Autodesk Inventor part; units mm, degrees
ref_plane "YZ Plane" through (0, 0, 0) normal (1, 0, 0) x (0, 1, 0)
ref_plane "XZ Plane" through (0, 0, 0) normal (0, 1, 0) x (-1, 0, 0)
ref_plane "XY Plane" through (0, 0, 0) normal (0, 0, 1) x (1, 0, 0)
sketch "Sketch1" plane through (0, 0, 0) normal (0, 0, 1) x (1, 0, 0)
  arc A0 (-20.5392, 17.1146) -> (-21.125, 15.7004) centre (-19.125, 15.7004) ccw
  line L0 (-21.125, -15.7004) -> (-21.125, 15.7004)
  arc A1 (-21.125, -15.7004) -> (-20.5392, -17.1146) centre (-19.125, -15.7004) ccw
  line L1 (-20.5392, -17.1146) -> (-17.1146, -20.5392)
  arc A2 (-17.1146, -20.5392) -> (-15.7004, -21.125) centre (-15.7004, -19.125) ccw
  line L2 (15.7004, -21.125) -> (-15.7004, -21.125)
  arc A3 (15.7004, -21.125) -> (17.1146, -20.5392) centre (15.7004, -19.125) ccw
  line L3 (20.5392, -17.1146) -> (17.1146, -20.5392)
  arc A4 (20.5392, -17.1146) -> (21.125, -15.7004) centre (19.125, -15.7004) ccw
  line L4 (21.125, 15.7004) -> (21.125, -15.7004)
  arc A5 (21.125, 15.7004) -> (20.5392, 17.1146) centre (19.125, 15.7004) ccw
  line L5 (20.5392, 17.1146) -> (17.1146, 20.5392)
  arc A6 (17.1146, 20.5392) -> (15.7004, 21.125) centre (15.7004, 19.125) ccw
  line L6 (-15.7004, 21.125) -> (15.7004, 21.125)
  arc A7 (-15.7004, 21.125) -> (-17.1146, 20.5392) centre (-15.7004, 19.125) ccw
  line L7 (-20.5392, 17.1146) -> (-17.1146, 20.5392)
  circle A8 centre (0, 0) radius 16
  circle A9 centre (-15.875, -15.875) radius 1.625
  circle A10 centre (15.875, 15.875) radius 1.625
  circle A11 centre (-15.875, 15.875) radius 1.625
  circle A12 centre (15.875, -15.875) radius 1.625
  circle A13 centre (0, 0) radius 12
  circle A14 centre (-15.875, 15.875) radius 2
  circle A15 centre (15.875, 15.875) radius 2
  circle A16 centre (15.875, -15.875) radius 2
  circle A17 centre (-15.875, -15.875) radius 2
  point P0 (0, 0)
  dimension "d0" = 24
  dimension "d1" = 4
  dimension "d2" = 4
  dimension "d3" = 4
  dimension "d4" = 4
extrude "Extrusion1" add sketch "Sketch1" along normal blind 5 contours L7 A7 L6 A6 L5 A5 L4 A4 L3 A3 L2 A2 L1 A1 L0 A0 | A8
sketch "Sketch3" plane through (0, 0, 5) normal (0, 0, 1) x (1, 0, 0)
  line L0 (-15.7004, 21.125) -> (15.7004, 21.125)
  line L1 (15.7004, 21.125) -> (-46.125, 21.125)
  line L2 (-46.125, 21.125) -> (-46.125, 26.125)
  line L3 (-46.125, 26.125) -> (15.7004, 26.125)
  line L4 (15.7004, 26.125) -> (15.7004, 21.125)
  line L5 (-21.125, 15.7004) -> (-21.125, -15.7004)
  line L6 (-21.125, -15.7004) -> (-26.125, -15.7004)
  line L7 (-26.125, -15.7004) -> (-26.125, 46.125)
  line L8 (-26.125, 46.125) -> (-21.125, 46.125)
  line L9 (-21.125, 46.125) -> (-21.125, -15.7004)
  point P0 (0, 0)
  dimension "d11" = 5
  dimension "d12" = 5
  dimension "d13" = 20
  dimension "d14" = 20
extrude "Extrusion3" add sketch "Sketch3" against normal blind 40
sketch "Sketch4" plane through (0, 0, 5) normal (0, 0, 1) x (1, 0, 0)
  arc A0 (-15.7004, 21.125) -> (-17.1146, 20.5392) centre (-15.7004, 19.125) ccw
  line L0 (-17.1146, 20.5392) -> (-20.5392, 17.1146)
  arc A1 (-20.5392, 17.1146) -> (-21.125, 15.7004) centre (-19.125, 15.7004) ccw
  line L1 (-21.125, 21.125) -> (-21.125, 15.7004)
  line L2 (-15.7004, 21.125) -> (-21.125, 21.125)
  circle A2 centre (0, 0) radius 12
  circle A3 centre (-15.875, -15.875) radius 2
  circle A4 centre (15.875, -15.875) radius 2
  circle A5 centre (15.875, 15.875) radius 2
  circle A6 centre (-15.875, 15.875) radius 2
  line L3 (15.7004, 26.125) -> (15.7004, 21.125)
  line L4 (-21.125, 26.125) -> (15.7004, 26.125)
  line L5 (-21.125, 46.125) -> (-21.125, 26.125)
  line L6 (-26.125, 46.125) -> (-21.125, 46.125)
  line L7 (-26.125, 26.125) -> (-26.125, 46.125)
  line L8 (-46.125, 26.125) -> (-26.125, 26.125)
  line L9 (-46.125, 21.125) -> (-46.125, 26.125)
  line L10 (-26.125, 21.125) -> (-46.125, 21.125)
  line L11 (-26.125, -15.7004) -> (-26.125, 21.125)
  line L12 (-21.125, -15.7004) -> (-26.125, -15.7004)
  arc A7 (-21.125, -15.7004) -> (-20.5392, -17.1146) centre (-19.125, -15.7004) ccw
  line L13 (-20.5392, -17.1146) -> (-17.1146, -20.5392)
  arc A8 (-17.1146, -20.5392) -> (-15.7004, -21.125) centre (-15.7004, -19.125) ccw
  line L14 (-15.7004, -21.125) -> (15.7004, -21.125)
  arc A9 (15.7004, -21.125) -> (17.1146, -20.5392) centre (15.7004, -19.125) ccw
  line L15 (17.1146, -20.5392) -> (20.5392, -17.1146)
  arc A10 (20.5392, -17.1146) -> (21.125, -15.7004) centre (19.125, -15.7004) ccw
  line L16 (21.125, -15.7004) -> (21.125, 15.7004)
  arc A11 (21.125, 15.7004) -> (20.5392, 17.1146) centre (19.125, 15.7004) ccw
  line L17 (20.5392, 17.1146) -> (17.1146, 20.5392)
  arc A12 (17.1146, 20.5392) -> (15.7004, 21.125) centre (15.7004, 19.125) ccw
  point P0 (0, 0)
extrude "Extrusion4" add sketch "Sketch4" against normal blind 5 contours A0 L0 A1 L1 L2
sketch "Sketch11" plane through (0, 0, 5) normal (0, 0, 1) x (1, 0, 0)
  line L0 (-26.125, 26.125) -> (-26.125, 46.125)
  line L1 (-26.125, 26.125) -> (-13.6996, 26.125)
  line L2 (-13.6996, 26.125) -> (-13.6996, 46.125)
  line L3 (-13.6996, 46.125) -> (-26.125, 46.125)
  line L4 (-26.125, 46.125) -> (-26.125, 26.125)
  line L5 (-46.125, 21.125) -> (-46.125, 26.125)
  line L6 (-46.125, 26.125) -> (-26.125, 26.125)
  line L7 (-26.125, 26.125) -> (-26.125, 13.3287)
  line L8 (-26.125, 13.3287) -> (-46.125, 13.3287)
  line L9 (-46.125, 13.3287) -> (-46.125, 26.125)
  point P0 (0, 0)
extrude "Extrusion9" cut sketch "Sketch11" against normal blind 20
sketch "Sketch7" plane through (0, 0, -35) normal (0, 0, -1) x (-1, 0, 0)
  line L0 (21.625, 21.625) -> (-23.2924, 21.625)
  line L1 (-23.2924, 21.625) -> (-23.2924, -21.9013)
  line L2 (-23.2924, -21.9013) -> (21.625, -21.9013)
  line L3 (21.625, -21.9013) -> (21.625, 21.625)
  line L4 (-15.7004, 21.125) -> (21.125, 21.125)
  line L5 (21.125, 21.125) -> (21.125, -15.7004)
  point P0 (0, 0)
  dimension "d35" = 0.5
  dimension "d36" = 0.5
extrude "Extrusion7" cut sketch "Sketch7" against normal blind 35
sketch "Sketch12" plane through (0, 0, -35) normal (0, 0, -1) x (-1, 0, 0)
  line L0 (46.125, 21.125) -> (46.125, 26.125)
  line L1 (26.125, 26.125) -> (-15.7004, 26.125)
  line L2 (46.125, 21.125) -> (21.6284, 21.125)
  line L3 (21.6284, 21.125) -> (21.6284, 26.125)
  line L4 (21.6284, 26.125) -> (46.125, 26.125)
  line L5 (46.125, 26.125) -> (46.125, 21.125)
  line L6 (26.125, 46.125) -> (21.125, 46.125)
  line L7 (-15.7004, 21.625) -> (21.625, 21.625)
  line L8 (26.125, 46.125) -> (21.125, 46.125)
  line L9 (21.125, 46.125) -> (21.125, 21.625)
  line L10 (21.125, 21.625) -> (26.125, 21.625)
  line L11 (26.125, 21.625) -> (26.125, 46.125)
  point P0 (0, 0)
  point P1 (21.125, 26.125)
  dimension "d54" = 5
  dimension "d55" = 5
  dimension "d56" = 4.5
  dimension "d57" = 0.5
extrude "Extrusion10" add sketch "Sketch12" along normal blind 20 contours L2 L3 L10 L11 L4 L0 | L11 L10 L3 L1 | L1 L9 L6 L11
sketch "Sketch13" plane through (-46.125, 21.125, -15) normal (0, -1, 0) x (1, 0, 0)
  circle A0 centre (10, -30) radius 2.5
  circle A1 centre (10, -10) radius 2.5
  line L0 (24.4966, -40) -> (0, -40)
  line L1 (0, 0) -> (0, -40)
  point P0 (46.125, 15)
  dimension "d60" = 10
  dimension "d61" = 10
  dimension "d62" = 5
  dimension "d63" = 5
  dimension "d64" = 20
  dimension "d65" = 10
extrude "Extrusion11" cut sketch "Sketch13" against normal blind 20
sketch "Sketch14" plane through (-26.125, 26.125, -15) normal (-1, 0, 0) x (0, 0, 1)
  circle A0 centre (-10, 10) radius 2.5
  circle A1 centre (-30, 10) radius 2.5
  line L0 (0, 0) -> (0, 20)
  line L1 (0, 20) -> (-40, 20)
  point P0 (15, -26.125)
  dimension "d68" = 10
  dimension "d69" = 10
  dimension "d70" = 20
  dimension "d71" = 10
  dimension "d72" = 5
  dimension "d73" = 5
extrude "Extrusion12" cut sketch "Sketch14" against normal blind 20
equation "\"d36\" = d35"
properties part number "StepperXYHolder"
Design review of the part built by this model. Coordinates are the model's own, in mm. A direction names the side the tool comes from. Round coordinates to 2 decimals unless told otherwise and drop trailing zeros. Order: outer loops, then holes, each group sorted by start corner. A loop starts at its lowest first (then second) coordinate and runs counter-clockwise, first axis right, second up.
1) Clearance check with flat-ended pins moving along their axes: pin 1 Ø3 at (y, z) = (6, -30) entering from -X (3 decimals); pin 2 Ø1.5 at (y, z) = (22.5, -10.5) entering from +X; pin 3 Ø6 at (x, z) = (-38.5, -26.5) entering from +Y (3 decimals); pin 4 Ø5 at (x, y) = (-34.5, 31) entering from -Z. State where each tip first meets the part, or that it passes through.
The answers:
pin 1: stops at x = -26.125
pin 2: stops at x = 15.7
pin 3: stops at y = 26.125
pin 4: passes through
2) Consider section C-C (x = 0). State the section outline as (y, z) points (3 decimals), plus the area to 3 significant figures.
The answers:
outline: (-21.125, 0) - (-12, 0) - (-12, 5) - (-21.125, 5) - close; (12, 0) - (21.625, 0) - (21.625, -35) - (26.125, -35) - (26.125, 5) - (12, 5) - close
area: 274 mm2
3) Consider section D-D (z = -45). State the section outline as (x, y) points (3 decimals).
The answers:
outline: (-46.125, 21.125) - (-38.625, 21.125) - (-38.625, 26.125) - (-46.125, 26.125) - close; (-33.625, 21.125) - (-21.628, 21.125) - (-21.628, 26.125) - (-21.125, 26.125) - (-21.125, 33.625) - (-26.125, 33.625) - (-26.125, 26.125) - (-33.625, 26.125) - close; (-26.125, 38.625) - (-21.125, 38.625) - (-21.125, 46.125) - (-26.125, 46.125) - close
4) Draft analysis for pull direction Y (two halves, no side actions). For faces 1 (the flat face through (18.851, 18.803, 2.465)), 2 (the flat face through (-21.125, 36, -35)), 3 (the flat face through (-24, -15.7, -15)), 4 (the cylindrical face through (-23.66, 35.17, -42.69)), state which applies: released by +Y, released by -Y, zero draft, split by the parting line, or undercut.
The answers:
face 1: released by +Y
face 2: zero draft
face 3: released by -Y
face 4: undercut
5) Machinability: for faces 5 (the flat face through (-21.625, 3, -18)), 6 (the flat face through (-24, 36, -15)), 7 (the flat face through (-36, 24, -15)), 8 (the flat face through (-26.125, 36, -35)), which of the approach directions +Z, -Z, +X, -X, +Y, -Y give a long, thin tool a straight path to every point of the face, cutting with its end or side? Answer none if there is none.
The answers:
face 5: -Z, +X, -Y
face 6: +Z, +X, -X, +Y
face 7: +Z, -X, +Y, -Y
face 8: +Z, -Z, -X, +Y
6) For L1, parallel to Y at x = -22.75, z = -45 (3 decimals); L2, parallel to Y at x = -31.5, z = -38 (3 decimals); L3, parallel to X at y = 42, z = -30.5 (3 decimals), list the stretches that pass through material, from the lowest coordinate up.
The answers:
L1: y = 21.125 to 33.625, 38.625 to 46.125
L2: y = 21.125 to 26.125
L3: x = -26.125 to -21.125
7) Consider section B-B (z = -25). State the section outline as (x, y) points (3 decimals).
The answers:
outline: (-46.125, 21.125) - (-38.625, 21.125) - (-38.625, 26.125) - (-46.125, 26.125) - close; (-33.625, 21.125) - (-26.125, 21.125) - (-26.125, -15.7) - (-21.625, -15.7) - (-21.625, 21.625) - (15.7, 21.625) - (15.7, 26.125) - (-21.125, 26.125) - (-21.125, 33.625) - (-26.125, 33.625) - (-26.125, 26.125) - (-33.625, 26.125) - close; (-26.125, 38.625) - (-21.125, 38.625) - (-21.125, 46.125) - (-26.125, 46.125) - close
8) Consider section A-A (y = 0). State the section outline as (x, z) points (3 decimals), plus the area to 3 significant figures.
The answers:
outline: (-26.125, -35) - (-21.625, -35) - (-21.625, 0) - (-12, 0) - (-12, 5) - (-26.125, 5) - close; (12, 0) - (21.125, 0) - (21.125, 5) - (12, 5) - close
area: 274 mm2
